```python
from build123d import *

# Parameters (mm, degrees)
CROQUIS1_W                = 300
CROQUIS1_H                = 50
SALIENTE_EXTRUIR1_DEPTH   = 2
CROQUIS2_R                = 6
CORTAR_EXTRUIR1_DEPTH     = 153.082214608
SIMETR_A2_COPY_1_SKETCH_R = 6
SIMETR_A2_COPY_1_DEPTH    = 153.082214608


with BuildPart() as part:
    # Croquis1 → Saliente-Extruir1 (new body)
    with BuildSketch(Plane.XY):
        Rectangle(CROQUIS1_W, CROQUIS1_H)
    extrude(amount=SALIENTE_EXTRUIR1_DEPTH)

    # Croquis2 → Cortar-Extruir1 (cut, through all)
    with BuildSketch(Plane.XY.offset(2)):
        with Locations((-140, -15)):
            Circle(CROQUIS2_R)
    cortar_extruir1 = extrude(amount=-CORTAR_EXTRUIR1_DEPTH, mode=Mode.SUBTRACT)

    # Simetría1: Cortar-Extruir1 across plane
    add(cortar_extruir1.mirror(Plane.ZX), mode=Mode.SUBTRACT)

    # Simetría2: Cortar-Extruir1 across plane
    add(cortar_extruir1.mirror(Plane(origin=(0, 0, 0), x_dir=(0, 0, 1), z_dir=(1, 0, 0))), mode=Mode.SUBTRACT)

    # Simetría2 copy 1 sketch → Simetría2 copy 1 (cut, through all)
    with BuildSketch(Plane(origin=(0, 0, 2), x_dir=(-1, 0, 0), z_dir=(0, 0, 1))):
        with Locations((-140, -15)):
            Circle(SIMETR_A2_COPY_1_SKETCH_R)
    extrude(amount=-SIMETR_A2_COPY_1_DEPTH, mode=Mode.SUBTRACT)


solid = part.part
```
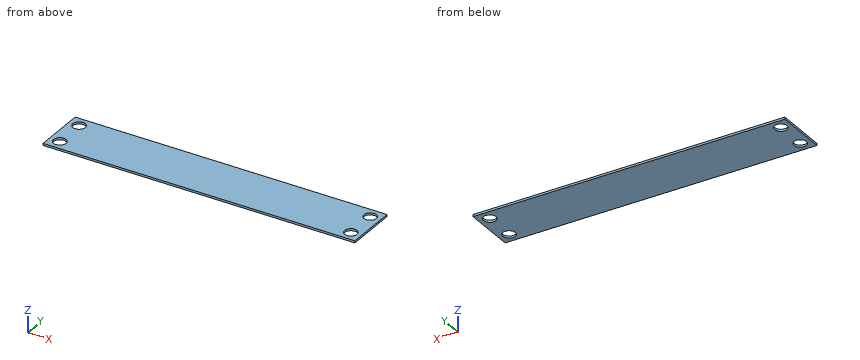
Model file for the job. Use its own axes, mm. Coordinates: 2 decimals unless noted, no trailing zeros. Order: outer loops, then holes, each group sorted by start corner. A loop starts at its lowest first (then second) coordinate and runs counter-clockwise, first axis right, second up. Notation, with made-up numbers: (-20, 57.25) - (35, 57.25) arc R13 cw to (35, 76.25) - close; hole circle Ø7 at (29, 59). An arc over 180 degrees is marked (long way). Return JSON: item names as keys, results as strings. Group by question number.
1) Saw through at A-A, the plane z = 1.55. Write the cut outline in (x, y).
2) Probe line 1 (Y direction, x = 140, z = 1.2); line 2 (X direction, y = 19, z = 1.2); line 3 (X direction, y = -10, z = 0.6). List the from-to ranges inside material, lowest first. Write a range as from..to.
3) Saw through at B-B, the plane y = -15. Write the cut outline in (x, z).
4) Saw through at C-C, the plane x = 140. Write the cut outline in (y, z), plus the area to 3 significant figures.
Values found:
{
 "1": {"outline": "(-150, -25) - (150, -25) - (150, 25) - (-150, 25) - close; hole circle Ø12 at (-140, -15); hole circle Ø12 at (-140, 15); hole circle Ø12 at (140, -15); hole circle Ø12 at (140, 15)"},
 "2": {"line 1": "y = -25..-21, -9..9, 21..25", "line 2": "x = -150..-144.47, -135.53..135.53, 144.47..150", "line 3": "x = -150..-143.32, -136.68..136.68, 143.32..150"},
 "3": {"outline": "(-150, 0) - (-146, 0) - (-146, 2) - (-150, 2) - close; (-134, 0) - (134, 0) - (134, 2) - (-134, 2) - close; (146, 0) - (150, 0) - (150, 2) - (146, 2) - close"},
 "4": {"outline": "(-25, 0) - (-21, 0) - (-21, 2) - (-25, 2) - close; (-9, 0) - (9, 0) - (9, 2) - (-9, 2) - close; (21, 0) - (25, 0) - (25, 2) - (21, 2) - close", "area": "52.0 mm²"}
}
